from build123d import *

# Parameters (mm, degrees)
SKETCH005_W  = 25
SKETCH005_H  = 80
PAD004_DEPTH = 3
SKETCH003_R  = 4
PAD002_DEPTH = 10
SKETCH004_W  = 40
SKETCH004_H  = 40
PAD003_DEPTH = 3
SKETCH006_W  = 25
SKETCH006_H  = 80
PAD005_DEPTH = 3


with BuildPart() as pad004:
    # Sketch005 → Pad004 (new body)
    with BuildSketch(Plane.XZ.offset(-12.5)):
        with Locations((-34, -50.041499)):
            Rectangle(SKETCH005_W, SKETCH005_H)
    extrude(amount=-PAD004_DEPTH)


with BuildPart() as pad002:
    # Sketch003 → Pad002 (new body)
    with BuildSketch(Plane(origin=(-12.5, 0, 0), x_dir=(0, -1, 0), z_dir=(-1, 0, 0))):
        with Locations((7.5, -25)):
            Circle(SKETCH003_R)
    extrude(amount=PAD002_DEPTH)


with BuildPart() as pad003:
    # Sketch004 → Pad003 (new body)
    with BuildSketch(Plane(origin=(-22.5, 0, 0), x_dir=(0, -1, 0), z_dir=(-1, 0, 0))):
        with Locations((7.5, -30)):
            Rectangle(SKETCH004_W, SKETCH004_H)
    extrude(amount=PAD003_DEPTH)


with BuildPart() as fusion005:
    # Sketch006 → Pad005 (new body)
    with BuildSketch(Plane.XZ.offset(27.5)):
        with Locations((-34, -50.041499)):
            Rectangle(SKETCH006_W, SKETCH006_H)
    extrude(amount=PAD005_DEPTH)

    # Fusion005: union Pad004, Pad002, Pad003
    add(pad004.part)
    add(pad002.part)
    add(pad003.part)


solid = fusion005.part
Can you work these out from the model? Positions are in its coordinate system, mm. A direction names the side the tool comes from. Coordinates: 2 decimals unless noted, no trailing zeros. Loops run counter-clockwise (first coordinate to the right, second up) from the corner with the lowest first, then second, coordinate; pieces in that order, holes last. Notation, with made-up numbers: M -16,58.5 L 12,58.5 A24 cw 12,76.5 Z; hole C 76.25,81.25 d11. An arc over 180 degrees is marked long. Return JSON: item names as keys, results as strings. Group by question number.
Item 1: If I drill on L1, parallel to Y at x = -31, z = -78.5; L2, parallel to X at y = 13.5, z = -24.5; L3, parallel to X at y = -24, z = -22.5, over which ranges is the centre line in solid material (lowest first)? Write a range as from..to.
Item 2: Imagine slicing it at B-B (x = -40.5). Please give me the cut outline in (y, z), and give its area (3 significant figures).
Item 3: On a 3-axis mill with a long thin cutter (end or side, diameter ignored), from which of +Z, -Z, +X, -X, +Y, -Y can I reach the whole of each face in a straight line? I mean faces 1 (the flat face through (-24, -7, -50)), 2 (the cylindrical face through (-17.43, -6.979, -21.034)), 3 (the flat face through (-46.5, 14, -51)). Say none if no direction works.
Item 4: Thinking about a two-plate mould opening in Y: for faces 4 (the flat face through (-24, -7, -10)), 5 (the flat face through (-25.5, -7, -30)), 6 (the flat face through (-34, 15.5, -49)), which applies, released by +Y, released by -Y, zero draft, split by the parting line, or undercut?
Item 5: I'm going to push flat-ended pins straight in: pin 1 Ø12 at (y, z) = (-5.5, -38) entering from -X; pin 2 Ø1.5 at (y, z) = (13.5, -54.5) entering from +X; pin 3 Ø5 at (y, z) = (-6.5, -33) entering from +X. Where does each tip first touch, or does it pass through?
Item 6: Imagine slicing it at C-C (y = -7.5). Please give me the cut outline in (x, z).
Item 7: Imagine slicing it at A-A (z = -53). Please give me the cut outline in (x, y), and give its area (3 significant figures).
Item 8: Imagine slicing it at D-D (z = -37.5). Please give me the cut outline in (x, y), and give its area (3 significant figures).
Verdict:
{
 "1": {"L1": "y = -30.5..-27.5, 12.5..15.5", "L2": "x = -46.5..-21.5", "L3": "x = -25.5..-22.5"},
 "2": {"outline": "M -30.5,-90.04 L -27.5,-90.04 L -27.5,-10.04 L -30.5,-10.04 Z; M 12.5,-90.04 L 15.5,-90.04 L 15.5,-10.04 L 12.5,-10.04 Z", "area": "480 mm^2"},
 "3": {"face 1": "-Z, +X, -X", "face 2": "+X", "face 3": "+Z, -Z, -X, +Y, -Y"},
 "4": {"face 4": "zero draft", "face 5": "undercut", "face 6": "released by +Y"},
 "5": {"pin 1": "stops at x = -25.5", "pin 2": "stops at x = -21.5", "pin 3": "stops at x = -22.5"},
 "6": {"outline": "M -25.5,-50 L -22.5,-50 L -22.5,-29 L -12.5,-29 L -12.5,-21 L -22.5,-21 L -22.5,-10 L -25.5,-10 Z"},
 "7": {"outline": "M -46.5,-30.5 L -21.5,-30.5 L -21.5,-27.5 L -46.5,-27.5 Z; M -46.5,12.5 L -21.5,12.5 L -21.5,15.5 L -46.5,15.5 Z", "area": "150 mm^2"},
 "8": {"outline": "M -46.5,-30.5 L -21.5,-30.5 L -21.5,-27.5 L -22.5,-27.5 L -22.5,12.5 L -21.5,12.5 L -21.5,15.5 L -46.5,15.5 L -46.5,12.5 L -25.5,12.5 L -25.5,-27.5 L -46.5,-27.5 Z", "area": "270 mm^2"}
}
